Geometry: final body of the model. Coordinates: model frame, mm. Give positions to 0.01 mm unless a question says otherwise; leave off trailing zeros. Loops run counter-clockwise (first coordinate to the right, second up) from the corner with the lowest first, then second, coordinate; pieces in that order, holes last. Notation, with made-up numbers: (-16, 42) - (20, 42) arc R30 cw to (20, 66) - close; hole circle Ø9 at (57.5, 16). An arc over 180 degrees is marked (long way). Use CSV: the item, a comma, the result in double quotes. Start each with the question number.
```python
from build123d import *

# Parameters (mm, degrees)
CROQUIS1_W              = 32
CROQUIS1_H              = 4
CROQUIS1_R              = 1
SALIENTE_EXTRUIR1_DEPTH = 4
CROQUIS2_R              = 1.6
CROQUIS2_R_2            = 0.75
CORTAR_EXTRUIR1_DEPTH   = 4


with BuildPart() as part:
    # Croquis1 → Saliente-Extruir1 (new body)
    with BuildSketch(Plane.XY):
        with Locations((16, 2)):
            Rectangle(CROQUIS1_W, CROQUIS1_H)
        with Locations((2, 2)):
            Circle(CROQUIS1_R, mode=Mode.SUBTRACT)
        with Locations(Location((30, 2, 0), (0, 0, 180))):
            Circle(CROQUIS1_R, mode=Mode.SUBTRACT)
    extrude(amount=SALIENTE_EXTRUIR1_DEPTH)

    # Croquis2 → Cortar-Extruir1 (cut)
    with BuildSketch(Plane.XZ):
        with Locations((2, 5)):
            Circle(CROQUIS2_R)
        with Locations(Location((13, 2, 0), (0, 0, 270))):
            Circle(CROQUIS2_R_2)
        with Locations(Location((10, 2, 0), (0, 0, 270))):
            Circle(CROQUIS2_R_2)
        with Locations(Location((7, 2, 0), (0, 0, 270))):
            Circle(CROQUIS2_R_2)
        with Locations(Location((25, 2, 0), (0, 0, 90))):
            Circle(CROQUIS2_R_2)
        with Locations(Location((22, 2, 0), (0, 0, 90))):
            Circle(CROQUIS2_R_2)
        with Locations(Location((19, 2, 0), (0, 0, 90))):
            Circle(CROQUIS2_R_2)
        with Locations((30, 5)):
            Circle(CROQUIS2_R)
        with Locations(Location((28, 2, 0), (0, 0, 90))):
            Circle(CROQUIS2_R_2)
        with Locations(Location((4, 2, 0), (0, 0, 270))):
            Circle(CROQUIS2_R_2)
    extrude(amount=-CORTAR_EXTRUIR1_DEPTH, mode=Mode.SUBTRACT)


solid = part.part
```
Item 1: Section C-C (z = 0.4). Output: boundary loops of the cut face in (x, y), plus the area to 3 significant figures.
Item 2: Section B-B (y = 3.7). Give the number of separate pieces and of enclosed holes in the cut face, plus the area to 3 significant figures.
Item 3: Section D-D (x = 30). Output: boundary loops of the cut face in (y, z), plus the area to 3 significant figures.
Item 4: Section A-A (x = 19). Output: boundary loops of the cut face in (y, z).
Item 5: Ray query, probe 1 along Z at (x, y) = (28, 1.35); probe 2 along Y at (x, z) = (30, 2.2); probe 3 along X at (y, z) = (1.6, 0.55). Return the intervals inside material, ascending.
Item 6: Mould query, pull axis Z, two halves, no side actions, for faces 1 (the cylindrical face through (31, 2, 2)), 2 (the flat face through (16, 2, 0)), 3 (the cylindrical face through (28.29, 1.97, 2.69)). Classes: pulls with the +Z half, pulls with the -Z half, needs draft (parallel to the pull), parting line crosses it, or undercut.
Outcome:
1,outline,"(0, 0) - (32, 0) - (32, 4) - (0, 4) - close; hole circle Ø2 at (2, 2); hole circle Ø2 at (30, 2)"
1,area,"122 mm2"
2,separate pieces,"1"
2,enclosed holes,"8"
2,area,"112 mm2"
3,outline,"(0, 0) - (1, 0) - (1, 3.4) - (0, 3.4) - close; (3, 0) - (4, 0) - (4, 3.4) - (3, 3.4) - close"
3,area,"6.80 mm2"
4,outline,"(0, 0) - (4, 0) - (4, 1.25) - (0, 1.25) - close; (0, 2.75) - (4, 2.75) - (4, 4) - (0, 4) - close"
5,probe 1,"z = 0 to 1.25, 2.75 to 4"
5,probe 2,"y = 0 to 1, 3 to 4"
5,probe 3,"x = 0 to 1.08, 2.92 to 29.08, 30.92 to 32"
6,face 1,"needs draft"
6,face 2,"pulls with the -Z half"
6,face 3,"undercut"
